Could you check a few things on this drawing? It's one solid part, dimensions in mm from its lowest x, y, z. A direction names the side the tool comes from. Round coordinates to 2 decimals unless told otherwise and drop trailing zeros. Loops run counter-clockwise (first coordinate to the right, second up) from the corner with the lowest first, then second, coordinate; pieces in that order, holes last. Notation, with made-up numbers: M 65,11.5 L 104,11.5 A24 ccw 104,34.5 Z; hole C 37,-31.5 d11. An arc over 180 degrees is marked long. Put each result on its own line as item: value. Start each with the question number.
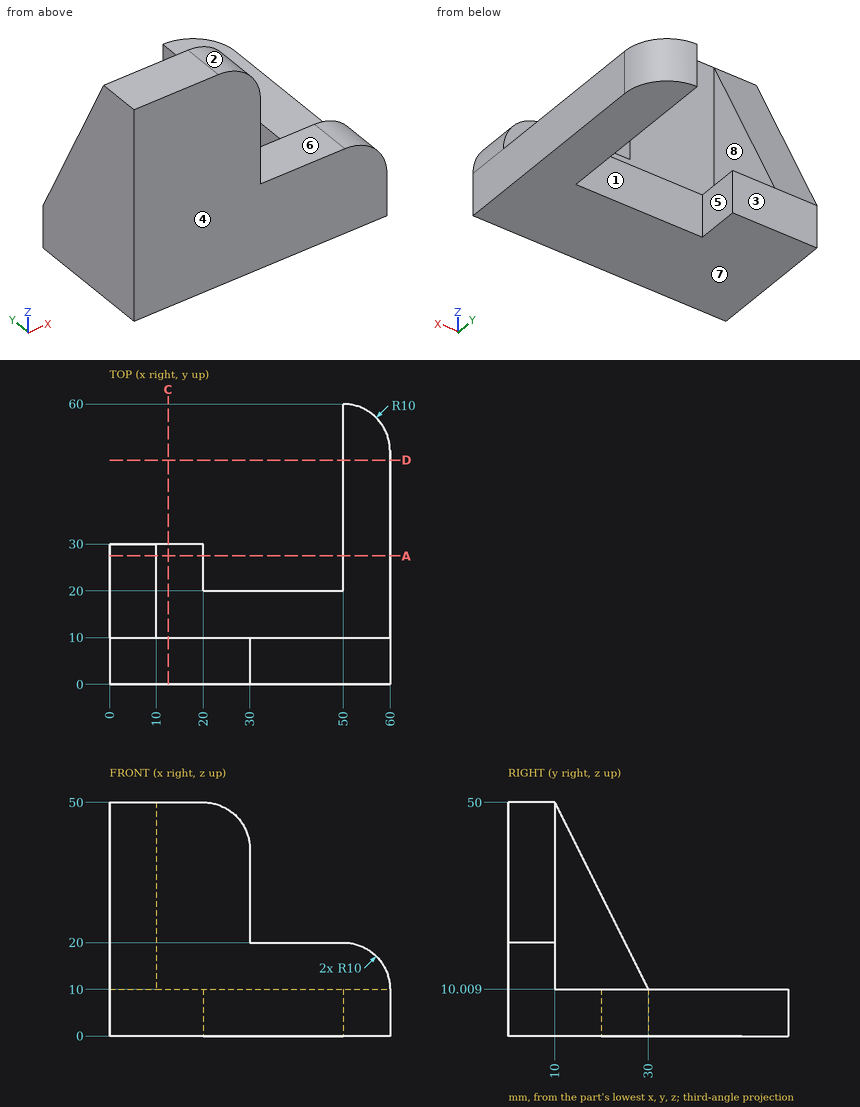
1) Suppose I cut it at A-A (y = 27.5). Write out the boundary of the cut face in (x, z), plus the area to 3 significant figures.
2) On a 3-axis mill with a long thin cutter (end or side, diameter ignored), from which of +Z, -Z, +X, -X, +Y, -Y can I reach the whole of each face in a straight line? I mean the marked faces 4, 5, 6, 7 and 8. Say none if no direction works.
3) Suppose I cut it at D-D (y = 48). Write out the boundary of the cut face in (x, z), plus the area to 3 significant figures.
4) If we mould it in two halves opening along X, with no side actions, what happens to the marked faces 1, 2 and 3? For each: pulls with the +X half, pulls with the -X half, needs draft (parallel to the pull), parting line crosses it, or undercut.
5) If I drill on probe 1 along Y at (x, z) = (23, 29); probe 2 along Y at (x, z) = (14, 9.5), over which ranges is the centre line in solid material (lowest first)? Write a range as from..to.
6) Suppose I cut it at C-C (x = 12.5). Write out the boundary of the cut face in (y, z), plus the area to 3 significant figures.
7) I'm going to push flat-ended pins straight in: P1, Ø3, axis at y = 40, z = 5, coming from the -X side; P2, Ø5, axis at x = 7.5, z = 3.5, coming from the +Y side; P3, Ø12, axis at x = 39, y = 18, coming from the +Z side; P4, Ø2, axis at x = 32, z = 44.5, coming from the -Y side. Where does each tip first touch, or does it pass through?
Results are:
1. outline: M 0,0 L 20,0 L 20,10 L 10,10 L 10,15.01 L 0,15.01 Z; M 50,0 L 60,0 L 60,10 L 50,10 Z
1. area: 350 mm²
2. face 4: +Z, -Z, +X, -X, -Y
2. face 5: +Z, -Z, +Y
2. face 6: +Z, +X, +Y, -Y
2. face 7: -Z, +X, -X, +Y, -Y
2. face 8: +Z, +X, +Y
3. outline: M 50,0 L 60,0 L 60,10 L 50,10 Z
3. area: 100 mm²
4. face 1: undercut
4. face 2: pulls with the +X half
4. face 3: needs draft
5. probe 1: 0..10
5. probe 2: 0..30
6. outline: M 0,0 L 30,0 L 30,10 L 10,10 L 10,50 L 0,50 Z
6. area: 700 mm²
7. P1: x = 50
7. P2: y = 30
7. P3: z = 10
7. P4: through
